from build123d import *

# Parameters (mm, degrees)
SKETCH1_R           = 40.005
BOSS_EXTRUDE1_DEPTH = 25.4
CUT_EXTRUDE1_REACH  = 64.016
SKETCH2_R           = 3.175
FILLET1_R           = 12.7


with BuildPart() as part:
    # Sketch1 → Boss-Extrude1 (new body)
    with BuildSketch(Plane.XY):
        Circle(SKETCH1_R)
    extrude(amount=BOSS_EXTRUDE1_DEPTH)

    # Sketch2 → Cut-Extrude1 (cut, up to next)
    with BuildSketch(Plane.XY.offset(25.4), mode=Mode.PRIVATE) as cut_extrude1_sk1:
        Circle(SKETCH2_R)
    cut_extrude1_tool1 = extrude(cut_extrude1_sk1.sketch, amount=-CUT_EXTRUDE1_REACH, mode=Mode.PRIVATE) & part.part
    add(cut_extrude1_tool1.solids().sort_by_distance((0, 0, 25.4))[0], mode=Mode.SUBTRACT)

    # Fillet1
    fillet1_edges = [part.edges().sort_by_distance(p)[0] for p in [
        (-40.005, 0, 0),
        (-40.005, 0, 25.4),
    ]]
    fillet(fillet1_edges, radius=FILLET1_R - 0.0001)  # a hair under: the kernel refuses the full size


solid = part.part
Input: part model. Units: mm. Frame: model coordinates. Round coordinates to 2 decimals unless told otherwise and drop trailing zeros. Loops run counter-clockwise (first coordinate to the right, second up) from the corner with the lowest first, then second, coordinate; pieces in that order, holes last. Notation, with made-up numbers: M 62,-31.5 L 85,-31.5 A38 cw 85,7.5 Z; hole C 80,-25 d11. An arc over 180 degrees is marked long. Answer as CSV lines item,"result". Start each with the question number.
(1) Line query: line 1 (Y direction, x = 0, z = 19.75) (3 decimals); line 2 (Y direction, x = 0, z = 14) (3 decimals); line 3 (Z direction, x = -4.5, y = -32). Output: solid intervals per line, ascending. Write a range as [from, to].
(2) Section C-C, the plane z = 3.25. Output: boundary loops of the cut face in (x, y) (3 decimals).
(3) Draft query along Y for faces 1 (the flat face through (0, -6, 25.4)), 2 (the cylindrical face through (-0.69, -3.1, 12.88)). Return one class per face: released by +Y, released by -Y, zero draft, split by the parting line, or undercut.
(4) Section D-D, the plane z = 23.5. Output: boundary loops of the cut face in (x, y) (3 decimals), plus the area to 3 significant figures.
(5) First-contact query: pin 1 (2 mm diameter, centred on x = 6, z = 17.5, fed in from -Y); pin 2 (2 mm diameter, centred on y = -17.5, z = 16.5, fed in from -X); pin 3 (1.5 mm diameter, centred on x = -5, z = 6, fed in from -Y); pin 4 (7.5 mm diameter, centred on x = 0, y = 0, fed in from +Z). Flat tips, straight axial feed; report the tip coordinate or a pass-through.
Values found:
1,line 1,"y = [-37.869, -3.175], [3.175, 37.869]"
1,line 2,"y = [-39.938, -3.175], [3.175, 39.938]"
1,line 3,"z = [1.03, 24.37]"
2,outline,"C 0,0 d71.579; hole C 0,0 d6.35"
3,face 1,"zero draft"
3,face 2,"undercut"
4,outline,"C 0,0 d67.974; hole C 0,0 d6.35"
4,area,"3,600 mm²"
5,pin 1,"stops at y = -39"
5,pin 2,"stops at x = -35.9"
5,pin 3,"stops at y = -38.21"
5,pin 4,"stops at z = 25.4"
